Can you work these out from the model? Positions are in its coordinate system, mm. A direction names the side the tool comes from. Round coordinates to 2 decimals unless told otherwise and drop trailing zeros. Write each loop counter-clockwise with the first axis right and the second up, starting at its lowest first coordinate (ties: lowest second). Pieces come first, ordered by that corner, then holes. Notation, with made-up numbers: M 43.25,86 L 92.25,86 A24 ccw 92.25,124 Z; hole C 0.25,-34 d4. An arc over 180 degrees is marked long. Answer as a JSON object with one key per item and string values. Group by question number.
1) I'm going to push flat-ended pins straight in: pin 1 Ø1.5 at (x, y) = (-28.5, 4) entering from +Z; pin 2 Ø5.5 at (x, z) = (-24.13, -19.05) entering from -Y; pin 3 Ø1.5 at (y, z) = (1.5, -8.5) entering from +X; pin 4 Ø1.4 at (x, y) = (-8, 2.5) entering from +Z. Where does each tip first touch, or does it pass through?
2) On a 3-axis mill with a long thin cutter (end or side, diameter ignored), from which of +Z, -Z, +X, -X, +Y, -Y can I reach the whole of each face in a straight line? I mean faces 4 (the flat face through (-12.7, 2, -7)), 5 (the cylindrical face through (-16.44, 2.415, -1.432)). Say none if no direction works.
3) Please list where these lines run through material, in increasing order: L1, parallel to Z at x = -24.13, y = 2.15 (3 decimals); L2, parallel to X at y = 4.5, z = -20; L3, parallel to X at y = 3.3, z = -19.05 (3 decimals). Write a range as [from, to].
4) Suppose I cut it at D-D, the plane z = -3.25. Write out the boundary of the cut face in (x, y).
5) If we mould it in two halves opening along Z, with no side actions, what happens to faces 1 (the flat face through (-14, 2, -1.27)), 2 (the cylindrical face through (-27.18, 2.35, -17.79)), 3 (the flat face through (-1.27, 2, -14))? For each: +Z half, -Z half, draft (parallel to the pull), parting line (faces both ways), or undercut.
6) Suppose I cut it at B-B, the plane z = -19.05. Write out the boundary of the cut face in (x, y) (1 decimal), and give its area (3 significant figures).
from build123d import *

# Parameters (mm, degrees)
BOSS_EXTRUDE1_DEPTH  = 4.7625
FILLET1_R            = 3.175
M6_CLEARANCE_HOLE1_D = 6.6


with BuildPart() as part:
    # Sketch1 → Boss-Extrude1 (new body)
    with BuildSketch(Plane(origin=(0, 0, 0), x_dir=(1, 0, 0), z_dir=(0, 1, 0))):
        with BuildLine():
            Line((-19.252221857, 27.231253289), (-1.27, 16.51))
            Line((-1.27, 16.51), (-1.27, 12.7))
            Line((-1.27, 12.7), (-12.7, 12.7))
            Line((-12.7, 12.7), (-12.7, 1.27))
            Line((-12.7, 1.27), (-16.51, 1.27))
            Line((-16.51, 1.27), (-29.902438631, 11.473419158))
            ThreePointArc((-29.902438631, 11.473419158), (-32.02160557, 24.383684142), (-19.252221857, 27.231253289))
        make_face()
    extrude(amount=BOSS_EXTRUDE1_DEPTH)

    # Fillet1
    fillet1_edges = [part.edges().sort_by_distance(p)[0] for p in [
        (-16.51, 2.38125, -1.27),
        (-1.27, 2.38125, -16.51),
    ]]
    fillet(fillet1_edges, radius=FILLET1_R)

    # M6 Clearance Hole1 (through all)
    with Locations(Plane(origin=(0, 4.7625, 0), x_dir=(1, 0, 0), z_dir=(0, 1, 0))):
        with Locations((-24.13, 19.05)):
            Hole(M6_CLEARANCE_HOLE1_D / 2)


solid = part.part
Results:
{
 "1": {"pin 1": "z = -9.83", "pin 2": "through", "pin 3": "x = -12.7", "pin 4": "z = -12.7"},
 "2": {"face 4": "+Z, +X, +Y, -Y", "face 5": "+Z, -X, +Y, -Y"},
 "3": {"L1": "[-28.575, -22.35], [-15.75, -7.076]", "L2": "[-33.61, -27.29], [-20.97, -7.12]", "L3": "[-33.655, -27.43], [-20.83, -5.53]"},
 "4": {"outline": "M -19.11,0 L -12.7,0 L -12.7,4.76 L -19.11,4.76 Z"},
 "5": {"face 1": "+Z half", "face 2": "undercut", "face 3": "draft"},
 "6": {"outline": "M -33.7,0 L -27.4,0 L -27.4,4.8 L -33.7,4.8 Z; M -20.8,0 L -5.5,0 L -5.5,4.8 L -20.8,4.8 Z", "area": "103 mm^2"}
}
